Work out the finished part from the listing and answer in its coordinate system (mm). Coordinates: 2 decimals unless noted, no trailing zeros. Order: outer loops, then holes, each group sorted by start corner. A loop starts at its lowest first (then second) coordinate and runs counter-clockwise, first axis right, second up. Notation, with made-up numbers: M 72.25,12.25 L 105.25,12.25 A6 ccw 105.25,16.25 Z; hole C 3,1 d5. An arc over 180 degrees is marked long. Write item = value, one per line. Start each with the question number.
Q1. Find section A-A on z = 1.1. Give the vertices of the cut face in (x, y) (3 decimals), and give its area (3 significant figures).
Q2. Determine the mould class of faces 1 (the flat face through (-39.531, 12, 1)), 2 (the cylindrical face through (-36.305, 34.744, 1.258)), 3 (the cylindrical face through (-35.725, -18.774, 1.252)) for opening direction Y: released by +Y, released by -Y, zero draft, split by the parting line, or undercut.
Q3. Straight lines are drawn through the part: line 1 along Y through (x, z) = (-35.5, 1.8); line 2 along Y through (x, z) = (-33.25, 1.1); line 3 along X through (y, z) = (38, 0.85). For each, find the intervals that lie inside material, in ascending order.
Q4. Find section B-B on x = -36.75. Give the number of separate pieces and of enclosed holes in the cut face, and give its area (3 significant figures).
Q5. Each of these flat-tipped pins is pushed along its axis until it touches: P1, Ø4, axis at x = -35.62, y = -14.85, coming from the -Z side; P2, Ø1.5, axis at x = -37, z = 1, coming from the -Y side. Where does it stop, or does it pass through?
```python
from build123d import *

# Parameters (mm, degrees)
F1_DEPTH = 2.54
F2_R     = 3.175
F2_R_2   = 3.171459
F3_DEPTH = 3.81
F4_R     = 0.381


with BuildPart() as f1:
    # F0 (on Top) → F1 (new body)
    with BuildSketch(Plane.XY):
        with BuildLine():
            ThreePointArc((-31.748279, 37.824634), (-35.639643, 41.715999), (-39.531007, 37.824634))
            Line((-39.531007, 37.824634), (-39.531007, -14.883377))
            ThreePointArc((-39.531007, -14.883377), (-35.639643, -18.774741), (-31.748279, -14.883377))
            Line((-31.748279, -14.883377), (-31.748279, 37.824634))
        make_face()
    extrude(amount=F1_DEPTH)

    # F2 (on Top) → F3 (cut)
    with BuildSketch(Plane.XY):
        with Locations((-35.616416, 37.843566)):
            Circle(F2_R)
        with Locations((-35.617653, -14.84884)):
            Circle(F2_R_2)
    extrude(amount=F3_DEPTH, mode=Mode.SUBTRACT)

    # F4
    f4_edges = [f1.edges().sort_by_distance(p)[0] for p in [
        (-38.791416, 37.843566, 2.54),
        (-38.791416, 37.843566, 0),
        (-38.789113, -14.84884, 2.54),
        (-38.789113, -14.84884, 0),
    ]]
    fillet(f4_edges, radius=F4_R)


solid = f1.part
```
Findings below:
q1.outline = M -39.531,-14.883 A3.891 ccw -31.748,-14.883 L -31.748,37.825 A3.891 ccw -39.531,37.825 Z; hole C -35.616,37.844 d6.35; hole C -35.618,-14.849 d6.343
q1.area = 395 mm^2
q2.face_1 = zero draft
q2.face_2 = undercut
q2.face_3 = released by -Y
q3.line_1 = -18.77 to -18.02, -11.68 to 34.67, 41.02 to 41.71
q3.line_2 = -17.95 to -16.96, -12.74 to 35.73, 39.96 to 40.9
q3.line_3 = -39.53 to -38.79, -32.45 to -31.75
q4.separate_pieces = 3
q4.enclosed_holes = 0
q4.area = 122 mm^2
q5.P1 = through
q5.P2 = -18.73
